The listing builds one solid part. Answer for the finished solid, in the listing's coordinates (mm). Give positions to 0.01 mm unless a question says otherwise; leave off trailing zeros. Write each loop counter-clockwise with the first axis right and the second up, starting at its lowest first coordinate (ties: lowest second). Pieces come first, ordered by that corner, then holes.
```python
from build123d import *

# Parameters (mm, degrees)
SKETCH1_R                                         = 21.5
SKETCH1_R_2                                       = 12
BOSS_EXTRUDE1_DEPTH                               = 2
SKETCH2_R                                         = 20
SKETCH2_R_2                                       = 13.6
BOSS_EXTRUDE2_DEPTH                               = 3
CHAMFER1_SIZE                                     = 1
CSK_FOR_0_FLAT_HEAD_MACHINE_SCREW_100_D           = 2.199999918
CSK_FOR_0_FLAT_HEAD_MACHINE_SCREW_100_CSINK_D     = 4.199999982
CSK_FOR_0_FLAT_HEAD_MACHINE_SCREW_100_CSINK_ANGLE = 100


with BuildPart() as part:
    # Sketch1 → Boss-Extrude1 (new body)
    with BuildSketch(Plane(origin=(0, 0, 0), x_dir=(1, 0, 0), z_dir=(0, 1, 0))):
        with Locations(Location((0, 0, 0), (0, 0, 270))):
            Circle(SKETCH1_R)
        with Locations(Location((0, 0, 0), (0, 0, 270))):
            Circle(SKETCH1_R_2, mode=Mode.SUBTRACT)
    extrude(amount=-BOSS_EXTRUDE1_DEPTH)

    # Sketch2 → Boss-Extrude2 (add)
    with BuildSketch(Plane.XZ.offset(2)):
        with Locations(Location((0, 0, 0), (0, 0, 270))):
            Circle(SKETCH2_R)
        with Locations(Location((0, 0, 0), (0, 0, 270))):
            Circle(SKETCH2_R_2, mode=Mode.SUBTRACT)
    extrude(amount=BOSS_EXTRUDE2_DEPTH)

    # Chamfer1
    chamfer1_edges = [part.edges().sort_by_distance(p)[0] for p in [
        (0, -5, 20),
    ]]
    chamfer(chamfer1_edges, length=CHAMFER1_SIZE)

    # CSK for #0 Flat Head Machine Screw (100)1 (through all)
    with Locations(Plane(origin=(0, 0, 0), x_dir=(1, 0, 0), z_dir=(0, 1, 0))):
        with Locations((0, 15), (12.990381057, -7.5), (-12.990381057, -7.5)):
            CounterSinkHole(CSK_FOR_0_FLAT_HEAD_MACHINE_SCREW_100_D / 2, CSK_FOR_0_FLAT_HEAD_MACHINE_SCREW_100_CSINK_D / 2, counter_sink_angle=CSK_FOR_0_FLAT_HEAD_MACHINE_SCREW_100_CSINK_ANGLE)


solid = part.part
```
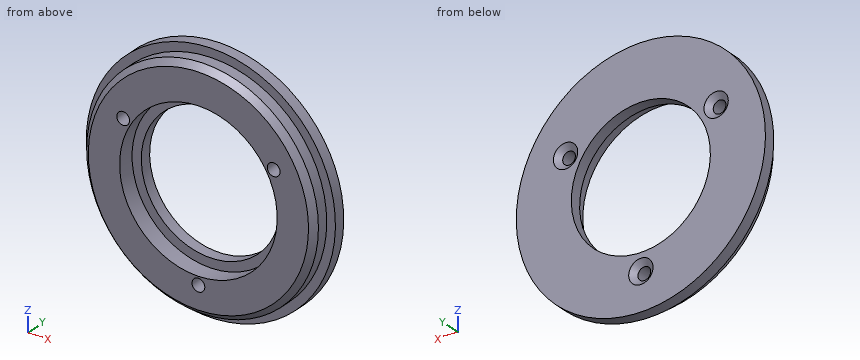
Item 1: A cutting plane is placed at B-B, the plane z = 7.5. Count the separate pieces of the cut face and the enclosed holes in it, plus the area to 3 significant figures.
Conclusion:
separate pieces: 4
enclosed holes: 0
area: 61.5 mm2
Item 2: Consider probe 1 along X at (y, z) = (-3.95, 7.5); probe 2 along X at (y, z) = (-1.2, 8.5); probe 3 along Z at (x, y) = (-12.5, -3.15). Determine where each line is inside the solid, lowest interval first.
Conclusion:
probe 1: x = -18.54 to -14.09, -11.89 to -11.35, 11.35 to 11.89, 14.09 to 18.54
probe 2: x = -19.75 to -13.45, -12.53 to -8.47, 8.47 to 12.53, 13.45 to 19.75
probe 3: z = -15.61 to -5.36, 5.36 to 6.52, 8.48 to 15.61
Item 3: A cutting plane is placed at A-A, the plane z = 0. Give the vertices of the cut face in (x, y), plus the area to 3 significant figures.
Conclusion:
outline: (-21.5, -2) - (-20, -2) - (-20, -4) - (-19, -5) - (-13.6, -5) - (-13.6, -2) - (-12, -2) - (-12, 0) - (-21.5, 0) - close; (12, -2) - (13.6, -2) - (13.6, -5) - (19, -5) - (20, -4) - (20, -2) - (21.5, -2) - (21.5, 0) - (12, 0) - close
area: 75.4 mm2
Item 4: Each of these flat-tipped pins is pushed along its axis until it touches: P1, Ø21.5, axis at x = 0, z = 0, coming from the -Y side; P2, Ø6, axis at x = 17, z = 0, coming from the +Y side; P3, Ø2, axis at x = 3, y = -2.5, coming from the -Z side; P4, Ø3.5, axis at x = -12.99, z = 7.5, coming from the +Y side. Where does it stop, or does it pass through?
Conclusion:
P1: passes through
P2: stops at y = 0
P3: stops at z = -21.39
P4: stops at y = -0.29
